```python
from build123d import *

# Parameters (mm, degrees)
SKETCH_1_R          = 17.5
EXTRUDE_1_DEPTH     = 50
SKETCH_3_R          = 18
EXTRUDE_4_DEPTH     = 35
SKETCH_4_R          = 8
EXTRUDE_5_DEPTH     = 2
SKETCH_5_R          = 3
EXTRUDE_6_DEPTH     = 22
SKETCH_6_R          = 1.5
CUT_EXTRUDE_1_DEPTH = 5
SKETCH_7_W          = 8.061647896
SKETCH_7_H          = 1.71902786
CUT_EXTRUDE_2_DEPTH = 18
FILLET_10_R         = 0.5
FILLET_11_R         = 0.5
FILLET_12_R         = 0.5
FILLET_13_R         = 0.5


with BuildPart() as part:
    # 草图1 → 凸台-拉伸1 (new body)
    with BuildSketch(Plane(origin=(0, 0, 0), x_dir=(1, 0, 0), z_dir=(0, 1, 0))):
        with Locations(Location((0, 0, 0), (0, 0, 270))):
            Circle(SKETCH_1_R)
    extrude(amount=EXTRUDE_1_DEPTH)

    # 草图3 → 凸台-拉伸4 (add)
    with BuildSketch(Plane(origin=(0, 50, 0), x_dir=(1, 0, 0), z_dir=(0, 1, 0))):
        with Locations(Location((0, 0, 0), (0, 0, 270))):
            Circle(SKETCH_3_R)
    extrude(amount=EXTRUDE_4_DEPTH)

    # 草图4 → 凸台-拉伸5 (add)
    with BuildSketch(Plane(origin=(0, 85, 0), x_dir=(1, 0, 0), z_dir=(0, 1, 0))):
        with Locations(Location((0, 0, 0), (0, 0, 270))):
            Circle(SKETCH_4_R)
    extrude(amount=EXTRUDE_5_DEPTH)

    # 草图5 → 凸台-拉伸6 (add)
    with BuildSketch(Plane(origin=(0, 87, 0), x_dir=(1, 0, 0), z_dir=(0, 1, 0))):
        with Locations(Location((0, 0, 0), (0, 0, 270))):
            Circle(SKETCH_5_R)
    extrude(amount=EXTRUDE_6_DEPTH)

    # 草图6 → 切除-拉伸1 (cut)
    with BuildSketch(Plane(origin=(0, 85, 0), x_dir=(1, 0, 0), z_dir=(0, 1, 0))):
        with Locations(Location((0, 12, 0), (0, 0, 270))):
            Circle(SKETCH_6_R)
        with Locations(Location((10.392304845, -6, 0), (0, 0, 270))):
            Circle(SKETCH_6_R)
        with Locations(Location((-10.392304845, -6, 0), (0, 0, 270))):
            Circle(SKETCH_6_R)
    extrude(amount=-CUT_EXTRUDE_1_DEPTH, mode=Mode.SUBTRACT)

    # 草图7 → 切除-拉伸2 (cut)
    with BuildSketch(Plane(origin=(0, 109, 0), x_dir=(1, 0, 0), z_dir=(0, 1, 0))):
        with Locations((-0.414937759, 2.85951393)):
            Rectangle(SKETCH_7_W, SKETCH_7_H)
    extrude(amount=-CUT_EXTRUDE_2_DEPTH, mode=Mode.SUBTRACT)

    # 圆角10
    fillet_10_edges = [part.edges().sort_by_distance(p)[0] for p in [
        (0, 85, -18),
    ]]
    fillet(fillet_10_edges, radius=FILLET_10_R)

    # 圆角11
    fillet_11_edges = [part.edges().sort_by_distance(p)[0] for p in [
        (0, 50, -18),
    ]]
    fillet(fillet_11_edges, radius=FILLET_11_R - 0.0001)  # a hair under: the kernel refuses the full size

    # 圆角12
    fillet_12_edges = [part.edges().sort_by_distance(p)[0] for p in [
        (0, 0, -17.5),
    ]]
    fillet(fillet_12_edges, radius=FILLET_12_R)

    # 圆角13
    fillet_13_edges = [part.edges().sort_by_distance(p)[0] for p in [
        (0, 87, -8),
    ]]
    fillet(fillet_13_edges, radius=FILLET_13_R)


solid = part.part
```
Work out the finished part from the listing and answer in its coordinate system (mm). A direction names the side the tool comes from. Coordinates: 2 decimals unless noted, no trailing zeros. Write each loop counter-clockwise with the first axis right and the second up, starting at its lowest first coordinate (ties: lowest second). Pieces come first, ordered by that corner, then holes.
Q1. Find the intervals of material crossed by line 1 (X direction, y = 82.75, z = 6); line 2 (Y direction, x = -10.5, z = -3.5); line 3 (Y direction, x = 7, z = -3), in increasing order.
Q2. A cutting plane is placed at D-D, the plane y = 20.5. Give the vertices of the cut face in (x, z).
Q3. Determine the mould class of faces 4 (the face through (-3.2, 87, -0.1)), 5 (the face through (-10.648, 24.904, -13.887)), 6 (the face through (-11.305, 82.535, 4.81)) for opening direction X: released by +X, released by -X, zero draft, split by the parting line, or undercut.
Q4. A cutting plane is placed at C-C, the plane y = 58. Give the vertices of the cut face in (x, z).
Q5. Which of the six approach directions +Z, -Z, +X, -X, +Y, -Y give full straight-line access (tool end or side, diameter ignored) to faces 1 (the face through (0.9, 97.85, 2.86)), 2 (the face through (0, 100, -2)), 3 (the face through (5.407, 67.262, 17.169))?
Q6. Each of these flat-tipped pins is pushed along its axis until it touches: pin 1 Ø3.5 at (x, y) = (0.5, 103) entering from -Z; pin 2 Ø6 at (y, z) = (74, -12.5) entering from +X; pin 3 Ø4 at (x, z) = (-10.39, 6) entering from +Y; pin 4 Ø4 at (x, z) = (0, -12) entering from -Y. Where does it stop, or does it pass through?
Findings below:
1. line 1: x = -16.97 to -11.89, -8.89 to 8.89, 11.89 to 16.97
1. line 2: y = 0 to 85
1. line 3: y = 0 to 86.99
2. outline: circle Ø35 at (0, 0)
3. face 4: zero draft
3. face 5: split by the parting line
3. face 6: undercut
4. outline: circle Ø36 at (0, 0)
5. face 1: +Y
5. face 2: -Z, +X, -X, +Y
5. face 3: +Y, -Y
6. pin 1: stops at z = -2
6. pin 2: stops at x = 15.29
6. pin 3: stops at y = 85
6. pin 4: stops at y = 0
